from build123d import *

# Parameters (mm, degrees)
SKETCH_1_W          = 50
SKETCH_1_H          = 20
EXTRUDE_1_DEPTH     = 3
SKETCH_2_W          = 50
SKETCH_2_H          = 12
EXTRUDE_2_DEPTH     = 6
SKETCH_5_W          = 50
SKETCH_5_H          = 9
CUT_EXTRUDE_2_DEPTH = 3
FILLET_1_R          = 4


with BuildPart() as part:
    # 草图1 → 凸台-拉伸1 (new body)
    with BuildSketch(Plane.XY):
        Rectangle(SKETCH_1_W, SKETCH_1_H)
        with BuildLine():
            Line((-3.85, 2.5), (3.85, 2.5))
            ThreePointArc((3.85, 2.5), (4.404700196, 2.667949706), (4.773076923, 3.115384615))
            ThreePointArc((4.773076923, 3.115384615), (20.35, 0), (4.773076923, -3.115384615))
            ThreePointArc((4.773076923, -3.115384615), (4.404700196, -2.667949706), (3.85, -2.5))
            Line((3.85, -2.5), (-3.85, -2.5))
            ThreePointArc((-3.85, -2.5), (-4.404700196, -2.667949706), (-4.773076923, -3.115384615))
            ThreePointArc((-4.773076923, -3.115384615), (-20.35, 0), (-4.773076923, 3.115384615))
            ThreePointArc((-4.773076923, 3.115384615), (-4.404700196, 2.667949706), (-3.85, 2.5))
        make_face(mode=Mode.SUBTRACT)
        with BuildLine():
            Line((3.25, 5.5), (-3.25, 5.5))
            ThreePointArc((-3.25, 5.5), (-5, 7.25), (-3.25, 9))
            Line((-3.25, 9), (3.25, 9))
            ThreePointArc((3.25, 9), (5, 7.25), (3.25, 5.5))
        make_face(mode=Mode.SUBTRACT)
    extrude(amount=EXTRUDE_1_DEPTH)

    # 草图2 → 凸台-拉伸2 (add)
    with BuildSketch(Plane(origin=(0, 10, 0), x_dir=(1, 0, 0), z_dir=(0, 1, 0))):
        with Locations((0, -6)):
            Rectangle(SKETCH_2_W, SKETCH_2_H)
    extrude(amount=EXTRUDE_2_DEPTH)

    # 草图5 → 切除-拉伸2 (cut)
    with BuildSketch(Plane.XZ.offset(-10)):
        with Locations((0, 7.5)):
            Rectangle(SKETCH_5_W, SKETCH_5_H)
    extrude(amount=-CUT_EXTRUDE_2_DEPTH, mode=Mode.SUBTRACT)

    # 圆角1
    fillet_1_edges = [part.edges().sort_by_distance(p)[0] for p in [
        (-25, 14.5, 12),
        (25, 14.5, 12),
        (25, -10, 1.5),
        (-25, -10, 1.5),
    ]]
    fillet(fillet_1_edges, radius=FILLET_1_R)


solid = part.part
The model under review builds one solid part; all positions refer to its coordinate system, in mm. A direction names the side the tool comes from. Round coordinates to 2 decimals unless told otherwise and drop trailing zeros. Write each loop counter-clockwise with the first axis right and the second up, starting at its lowest first coordinate (ties: lowest second). Pieces come first, ordered by that corner, then holes. Notation, with made-up numbers: (59, 65) -> (97, 65) arc R18 ccw to (97, 98) -> close; hole circle Ø7 at (-39, 42). An arc over 180 degrees is marked (long way). Answer as a JSON object with one key per item and string values.
1. We need section D-D on y = 3.75. State the section outline as (x, z) points.
Results found:
{"outline": "(-25, 0) -> (-19.43, 0) -> (-19.43, 3) -> (-25, 3) -> close; (-5.07, 0) -> (5.07, 0) -> (5.07, 3) -> (-5.07, 3) -> close; (19.43, 0) -> (25, 0) -> (25, 3) -> (19.43, 3) -> close"}
2. The part is to be moulded in two halves that separate along Y. For faces 4 (the face through (23.859, -8.797, 1.521)), 5 (the face through (0, 9, 1)), 6 (the face through (-23.859, 14.521, 10.797)), say which applies: pulls with the +Y half, pulls with the -Y half, needs draft (parallel to the pull), parting line crosses it, or undercut.
Results found:
{"face 4": "pulls with the -Y half", "face 5": "undercut", "face 6": "needs draft"}
3. Machinability: for faces 1 (the face through (0, 4, 3)), 2 (the face through (4.398, 2.663, 1.479)), 3 (the face through (23.859, 14.521, 10.797)), which of the approach directions +Z, -Z, +X, -X, +Y, -Y give a long, thin tool a straight path to every point of the face, cutting with its end or side? Answer none if there is none.
Results found:
{"face 1": "+Z, +X, -X, -Y", "face 2": "+Z, -Z", "face 3": "+Z, +X, +Y, -Y"}
4. Clearance check with flat-ended pins moving along their axes: pin 1 (10 mm diameter, centred on x = 14.5, y = 6.5, fed in from +Z); pin 2 (4 mm diameter, centred on x = -9.5, y = 4, fed in from -Z). State where each tip first meets the part, or that it passes through.
Results found:
{"pin 1": "stops at z = 3", "pin 2": "passes through"}
5. We need section B-B on x = 12.25. State the section outline as (y, z) points, and give its area (3 significant figures).
Results found:
{"outline": "(-10, 0) -> (-8.1, 0) -> (-8.1, 3) -> (-10, 3) -> close; (8.1, 0) -> (16, 0) -> (16, 12) -> (13, 12) -> (13, 3) -> (8.1, 3) -> close", "area": "56.4 mm^2"}
6. To check wall thickness, follow line 1 along Y through (x, z) = (-12.25, 2.2); line 2 along Y through (x, z) = (1.5, 1); line 3 along X through (y, z) = (4.25, 2). State the ranges of each line that lie inside material, in increasing order.
Results found:
{"line 1": "y = -10 to -8.1, 8.1 to 16", "line 2": "y = -10 to -2.5, 2.5 to 5.5, 9 to 16", "line 3": "x = -25 to -19.15, -5.35 to 5.35, 19.15 to 25"}
7. We need section C-C on z = 1.75. State the section outline as (x, y) points.
Results found:
{"outline": "(-25, -6) arc R4 ccw to (-21, -10) -> (21, -10) arc R4 ccw to (25, -6) -> (25, 16) -> (-25, 16) -> close; hole (-4.77, -3.12) arc R1 cw to (-3.85, -2.5) -> (3.85, -2.5) arc R1 cw to (4.77, -3.12) arc R8.1 ccw (long way) to (4.77, 3.12) arc R1 cw to (3.85, 2.5) -> (-3.85, 2.5) arc R1 cw to (-4.77, 3.12) arc R8.1 ccw (long way) to start; hole (-3.25, 5.5) -> (3.25, 5.5) arc R1.75 ccw to (3.25, 9) -> (-3.25, 9) arc R1.75 ccw to start"}
8. We need section A-A on y = 0. State the section outline as (x, z) points.
Results found:
{"outline": "(-25, 0) -> (-20.35, 0) -> (-20.35, 3) -> (-25, 3) -> close; (20.35, 0) -> (25, 0) -> (25, 3) -> (20.35, 3) -> close"}
